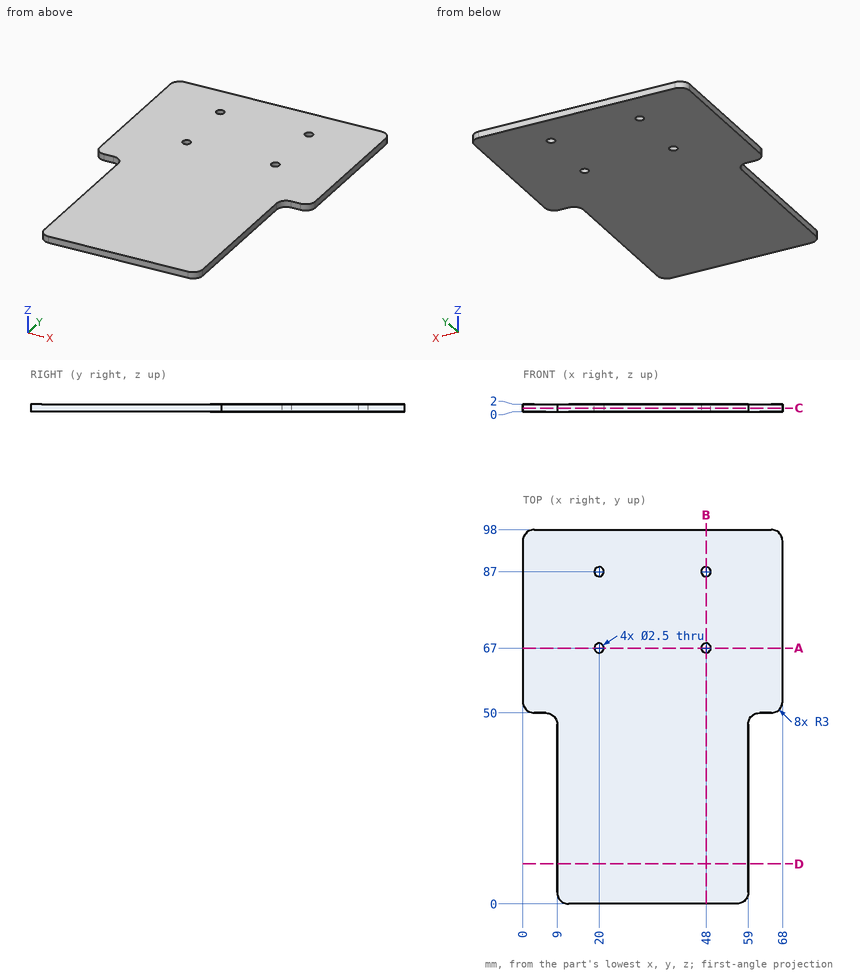
Design review of the part shown in the three views and the two pictorial views. Dimensions are in mm from the part's minimum x, y and z. Round coordinates to 2 decimals unless told otherwise and drop trailing zeros. Write each loop counter-clockwise with the first axis right and the second up, starting at its lowest first coordinate (ties: lowest second). Pieces come first, ordered by that corner, then holes.
Item 1: For pin 1 Ø1 at (x, y) = (18.5, 23.5) entering from -Z; pin 2 Ø0.6 at (x, z) = (63.5, 1.5) entering from -Y, all flat-tipped, find the tip position at first contact; note any pin that passes through.
Item 2: Consider section A-A on y = 67. Give the boundary of the cut face in (x, z), and give its area (3 significant figures).
Item 3: Consider section D-D on y = 10.5. Give the boundary of the cut face in (x, z), and give its area (3 significant figures).
Item 4: Wall thickness on L1, parallel to X at y = 87, z = 0.9; L2, parallel to Y at x = 48, z = 0.6; L3, parallel to X at y = 88, z = 1.1: over which ranges is each line inside the solid? List them lowest first.
Item 5: Consider section C-C on z = 0.9. Give the boundary of the cut face in (x, y).
Item 6: Consider section B-B on x = 48. Give the boundary of the cut face in (y, z), and give its area (3 significant figures).
Check values:
1. pin 1: stops at z = 0
1. pin 2: stops at y = 50
2. outline: (0, 0) - (18.75, 0) - (18.75, 2) - (0, 2) - close; (21.25, 0) - (46.75, 0) - (46.75, 2) - (21.25, 2) - close; (49.25, 0) - (68, 0) - (68, 2) - (49.25, 2) - close
2. area: 126 mm2
3. outline: (9, 0) - (59, 0) - (59, 2) - (9, 2) - close
3. area: 100 mm2
4. L1: x = 0 to 18.75, 21.25 to 46.75, 49.25 to 68
4. L2: y = 0 to 65.75, 68.25 to 85.75, 88.25 to 98
4. L3: x = 0 to 19.25, 20.75 to 47.25, 48.75 to 68
5. outline: (0, 53) arc R3 ccw to (3, 50) - (6, 50) arc R3 cw to (9, 47) - (9, 3) arc R3 ccw to (12, 0) - (56, 0) arc R3 ccw to (59, 3) - (59, 47) arc R3 cw to (62, 50) - (65, 50) arc R3 ccw to (68, 53) - (68, 95) arc R3 ccw to (65, 98) - (3, 98) arc R3 ccw to (0, 95) - close; hole circle Ø2.5 at (20, 67); hole circle Ø2.5 at (20, 87); hole circle Ø2.5 at (48, 67); hole circle Ø2.5 at (48, 87)
6. outline: (0, 0) - (65.75, 0) - (65.75, 2) - (0, 2) - close; (68.25, 0) - (85.75, 0) - (85.75, 2) - (68.25, 2) - close; (88.25, 0) - (98, 0) - (98, 2) - (88.25, 2) - close
6. area: 186 mm2
